Work out the finished part from the listing and answer in its coordinate system (mm). Face numbers are marked on the shaded views. A direction names the side the tool comes from. Coordinates: 2 decimals unless noted, no trailing zeros. Loops run counter-clockwise (first coordinate to the right, second up) from the corner with the lowest first, then second, coordinate; pieces in that order, holes last. Notation, with made-up numbers: (21, -36) - (57, -36) arc R28 cw to (57, -12) - close; hole circle Ø11 at (-21.75, 13). An arc over 180 degrees is marked (long way). Write each question's results on one line, items separated by ' | '. Start each with the question number.
1. A cutting plane is placed at C-C on x = 12.5. Determine the outline of the cut face in (y, z).
2. A cutting plane is placed at D-D on y = 14.75. Determine the outline of the cut face in (x, z), then the cut area to 3 significant figures.
3. Each of these flat-tipped pins is pushed along its axis until it touches: P1, Ø3.5, axis at x = 12, z = 14, coming from the -Y side; P2, Ø1, axis at x = -3.5, y = 15, coming from the -Z side; P3, Ø2.5, axis at x = 16, z = -1.5, coming from the +Y side; P4, Ø1, axis at x = 9.5, y = 18, coming from the +Z side. Where does it stop, or does it pass through?
4. Which of the six approach directions +Z, -Z, +X, -X, +Y, -Y give full straight-line access (tool end or side, diameter ignored) to the marked faces 4, 5, 6 and 7?
5. Determine the mould class of the marked faces 1, 2 and 3 for opening direction X: released by +X, released by -X, zero draft, split by the parting line, or undercut.
6. A cutting plane is placed at B-B on z = 13.5. Determine the outline of the cut face in (x, y), then the cut area to 3 significant figures.
7. A cutting plane is placed at A-A on x = 4. Determine the outline of the cut face in (y, z).
8. Find the intervals of material crossed by line 1 along X through (y, z) = (18.75, 12.5); line 2 along X through (y, z) = (6.75, 11); line 3 along Y through (x, z) = (5, 1.25), in increasing order. Write a range as [from, to].
from build123d import *

# Parameters (mm, degrees)
FLANGE_BASE1_DEPTH             = 3
CORTE_EXTRUS_O1_DEPTH          = 3
ARESTA_FLANGE4_STRIP_W         = 13.4732
ARESTA_FLANGE4_STRIP_H         = 3
ARESTA_FLANGE4_STRIP_CUT_DEPTH = 17.5
ARESTA_FLANGE4_DEPTH           = 17.5
ESBO_O47_W                     = 14.5
ESBO_O47_H                     = 15
RESSALTO_EXTRUS_O1_DEPTH       = 3
FILETE1_R                      = 5
ESBO_O48_W                     = 14.5
ESBO_O48_H                     = 15
RESSALTO_EXTRUS_O2_DEPTH       = 3
FILETE2_R                      = 5
FILETE3_R                      = 2
CORTE_EXTRUS_O5_DEPTH          = 42.11835661
CORTE_EXTRUS_O6_DEPTH          = 3


# Sheet-metal steps are written as plain solids
with BuildPart() as part:
    # Esboço1 → Flange-base1 (new body)
    with BuildSketch(Plane.XY):
        Polygon((-14.370772566, 2.693459119), (-4.370772566, 2.693459119), (-4.370772566, 5.693459119), (13.129227434, 5.693459119), (13.129227434, 2.693459119), (20.129227434, 2.693459119), (20.129227434, -4.306540881), (-14.370772566, -4.306540881), align=None)
    extrude(amount=-FLANGE_BASE1_DEPTH)

    # Esboço8 → Corte-extrusão1 (cut)
    with BuildSketch(Plane.XY):
        with BuildLine():
            Line((-10.260200759, 1.193459119), (-2.260200759, 1.193459119))
            ThreePointArc((-2.260200759, 1.193459119), (-0.260200759, -0.806540881), (-2.260200759, -2.806540881))
            Line((-2.260200759, -2.806540881), (-10.260200759, -2.806540881))
            ThreePointArc((-10.260200759, -2.806540881), (-12.260200759, -0.806540881), (-10.260200759, 1.193459119))
        make_face()
        with BuildLine():
            Line((8.88097681, 1.193459119), (17.620096532, 1.193459119))
            ThreePointArc((17.620096532, 1.193459119), (19.620096532, -0.806540881), (17.620096532, -2.806540881))
            Line((17.620096532, -2.806540881), (8.88097681, -2.806540881))
            ThreePointArc((8.88097681, -2.806540881), (6.88097681, -0.806540881), (8.88097681, 1.193459119))
        make_face()
    extrude(amount=-CORTE_EXTRUS_O1_DEPTH, mode=Mode.SUBTRACT)

    # Aresta-Flange4 strip (across the edge) → Aresta-Flange4 strip cut (cut)
    with BuildSketch(Plane(origin=(13.129227434, 5.693459119, 0), x_dir=(0, -1, 0), z_dir=(-1, 0, 0))):
        with Locations((-6, -1.5)):
            Rectangle(ARESTA_FLANGE4_STRIP_W, ARESTA_FLANGE4_STRIP_H)
    extrude(amount=ARESTA_FLANGE4_STRIP_CUT_DEPTH, mode=Mode.SUBTRACT)

    # Aresta-Flange4 section (across the edge) → Aresta-Flange4 (add)
    with BuildSketch(Plane(origin=(13.129227434, 5.693459119, 0), x_dir=(0, -1, 0), z_dir=(-1, 0, 0))):
        with BuildLine():
            Line((-3, 0.7366), (-3, 22.5))
            Line((-3, 22.5), (0, 22.5))
            Line((0, 22.5), (0, 0.7366))
            ThreePointArc((0, 0.7366), (0.215745145, 0.215745145), (0.7366, 0))
            Line((0.7366, 0), (0.7366, -3))
            ThreePointArc((0.7366, -3), (-1.905575199, -1.905575199), (-3, 0.7366))
        make_face()
    extrude(amount=ARESTA_FLANGE4_DEPTH)

    # Esboço47 → Ressalto-extrusão1 (add)
    with BuildSketch(Plane(origin=(13.129227434, 0, 0), x_dir=(0, 0, -1), z_dir=(1, 0, 0))):
        with Locations((-15.25, 13.193459119)):
            Rectangle(ESBO_O47_W, ESBO_O47_H)
    extrude(amount=-RESSALTO_EXTRUS_O1_DEPTH)

    # Filete1
    filete1_edges = [part.edges().sort_by_distance(p)[0] for p in [
        (11.629227434, 20.693459119, 22.5),
        (11.629227434, 8.693459119, 8),
        (11.629227434, 20.693459119, 8),
    ]]
    fillet(filete1_edges, radius=FILETE1_R)

    # Esboço48 → Ressalto-extrusão2 (add)
    with BuildSketch(Plane.ZY.offset(4.370772566)):
        with Locations((15.25, 13.193459119)):
            Rectangle(ESBO_O48_W, ESBO_O48_H)
    extrude(amount=-RESSALTO_EXTRUS_O2_DEPTH)

    # Filete2
    filete2_edges = [part.edges().sort_by_distance(p)[0] for p in [
        (-2.870772566, 20.693459119, 22.5),
        (-2.870772566, 8.693459119, 8),
        (-2.870772566, 20.693459119, 8),
    ]]
    fillet(filete2_edges, radius=FILETE2_R)

    # Filete3
    filete3_edges = [part.edges().sort_by_distance(p)[0] for p in [
        (20.129227434, -4.306540881, -1.5),
        (-14.370772566, -4.306540881, -1.5),
        (-14.370772566, 2.693459119, -1.5),
        (-4.370772566, 2.693459119, -1.5),
        (13.129227434, 2.693459119, -1.5),
        (20.129227434, 2.693459119, -1.5),
    ]]
    fillet(filete3_edges, radius=FILETE3_R)

    # Esboço49 → Corte-extrusão5 (cut, through all)
    with BuildSketch(Plane(origin=(13.129227434, 0, 0), x_dir=(0, 0, -1), z_dir=(1, 0, 0))):
        with BuildLine():
            Line((-18, 11.175198381), (-12.5, 11.175198381))
            ThreePointArc((-12.5, 11.175198381), (-11.085786438, 11.760984819), (-10.5, 13.175198381))
            Line((-10.5, 13.175198381), (-10.5, 16.193459119))
            ThreePointArc((-10.5, 16.193459119), (-11.085786438, 17.607672682), (-12.5, 18.193459119))
            Line((-12.5, 18.193459119), (-18, 18.193459119))
            ThreePointArc((-18, 18.193459119), (-19.414213562, 17.607672682), (-20, 16.193459119))
            Line((-20, 16.193459119), (-20, 13.175198381))
            ThreePointArc((-20, 13.175198381), (-19.414213562, 11.760984819), (-18, 11.175198381))
        make_face()
    extrude(amount=-CORTE_EXTRUS_O5_DEPTH, mode=Mode.SUBTRACT)

    # Esboço50 → Corte-extrusão6 (cut)
    with BuildSketch(Plane.XZ.offset(-5.693459119)):
        with BuildLine():
            Line((1.629227434, 19.2366), (7.129227434, 19.2366))
            ThreePointArc((7.129227434, 19.2366), (8.543440996, 18.650813562), (9.129227434, 17.2366))
            Line((9.129227434, 17.2366), (9.129227434, 5.2366))
            ThreePointArc((9.129227434, 5.2366), (8.543440996, 3.822386438), (7.129227434, 3.2366))
            Line((7.129227434, 3.2366), (1.629227434, 3.2366))
            ThreePointArc((1.629227434, 3.2366), (0.215013871, 3.822386438), (-0.370772566, 5.2366))
            Line((-0.370772566, 5.2366), (-0.370772566, 17.2366))
            ThreePointArc((-0.370772566, 17.2366), (0.215013871, 18.650813562), (1.629227434, 19.2366))
        make_face()
    extrude(amount=-CORTE_EXTRUS_O6_DEPTH, mode=Mode.SUBTRACT)


solid = part.part
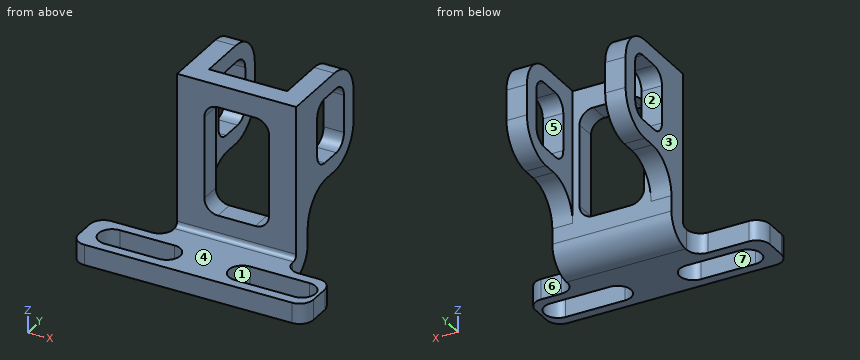
Values:
1) outline: (-4.31, -3) - (-2.81, -3) - (-2.81, 0) - (-4.31, 0) - close; (1.19, -3) - (4.96, -3) arc R3.74 ccw to (8.69, 0.74) - (8.69, 3) arc R5 cw to (13.69, 8) - (15.69, 8) arc R5 ccw to (20.69, 13) - (20.69, 17.5) arc R5 ccw to (15.69, 22.5) - (5.69, 22.5) - (5.69, 0.74) arc R0.74 cw to (4.96, 0) - (1.19, 0) - close; hole (11.18, 12.5) arc R2 ccw to (13.18, 10.5) - (16.19, 10.5) arc R2 ccw to (18.19, 12.5) - (18.19, 18) arc R2 ccw to (16.19, 20) - (13.18, 20) arc R2 ccw to (11.18, 18) - close
2) outline: (-4.37, 8) - (-1.37, 8) - (-1.37, 10.5) - (-4.37, 10.5) - close; (-4.37, 20) - (-1.37, 20) - (-1.37, 22.5) - (-4.37, 22.5) - close; (10.13, 8) - (13.13, 8) - (13.13, 10.5) - (10.13, 10.5) - close; (10.13, 20) - (13.13, 20) - (13.13, 22.5) - (10.13, 22.5) - close | area: 30.0 mm^2
3) P1: y = 5.69 | P2: z = 8 | P3: y = 2.73 | P4: through
4) face 4: +Z, +X, -X, -Y | face 5: +X, -X | face 6: +Z, -Z, +X, +Y | face 7: +Z, -Z
5) face 1: undercut | face 2: zero draft | face 3: released by -X
6) outline: (-4.37, 5.69) - (-0.37, 5.69) - (-0.37, 8.69) - (-1.37, 8.69) - (-1.37, 11.18) - (-4.37, 11.18) - close; (-4.37, 18.19) - (-1.37, 18.19) - (-1.37, 20.69) - (-4.37, 20.69) - close; (9.13, 5.69) - (13.13, 5.69) - (13.13, 11.18) - (10.13, 11.18) - (10.13, 8.69) - (9.13, 8.69) - close; (10.13, 18.19) - (13.13, 18.19) - (13.13, 20.69) - (10.13, 20.69) - close | area: 53.9 mm^2
7) outline: (-4.31, -3) - (4.96, -3) arc R3.74 ccw to (8.69, 0.74) - (8.69, 3.24) - (5.69, 3.24) - (5.69, 0.74) arc R0.74 cw to (4.96, 0) - (-4.31, 0) - close; (5.69, 19.24) - (8.69, 19.24) - (8.69, 22.5) - (5.69, 22.5) - close
8) line 1: [-4.37, -1.37], [10.13, 13.13] | line 2: [-4.37, -0.37], [9.13, 13.13] | line 3: [5.69, 8.69]
